Source: three-view drawing plus pictorial views. Frame: mm from the lowest corner of the part. A direction names the side the tool comes from. Give positions to 0.01 mm unless a question says otherwise; leave off trailing zeros. Order: outer loops, then holes, each group sorted by start corner. A loop starts at its lowest first (then second) coordinate and runs counter-clockwise, first axis right, second up. Notation, with made-up numbers: M 74.25,78.5 L 85.25,78.5 A24 ccw 85.25,92.5 Z; hole C -23.75,6.25 d9. An arc over 180 degrees is marked long. Use CSV: the item, a comma, the result in double quotes.
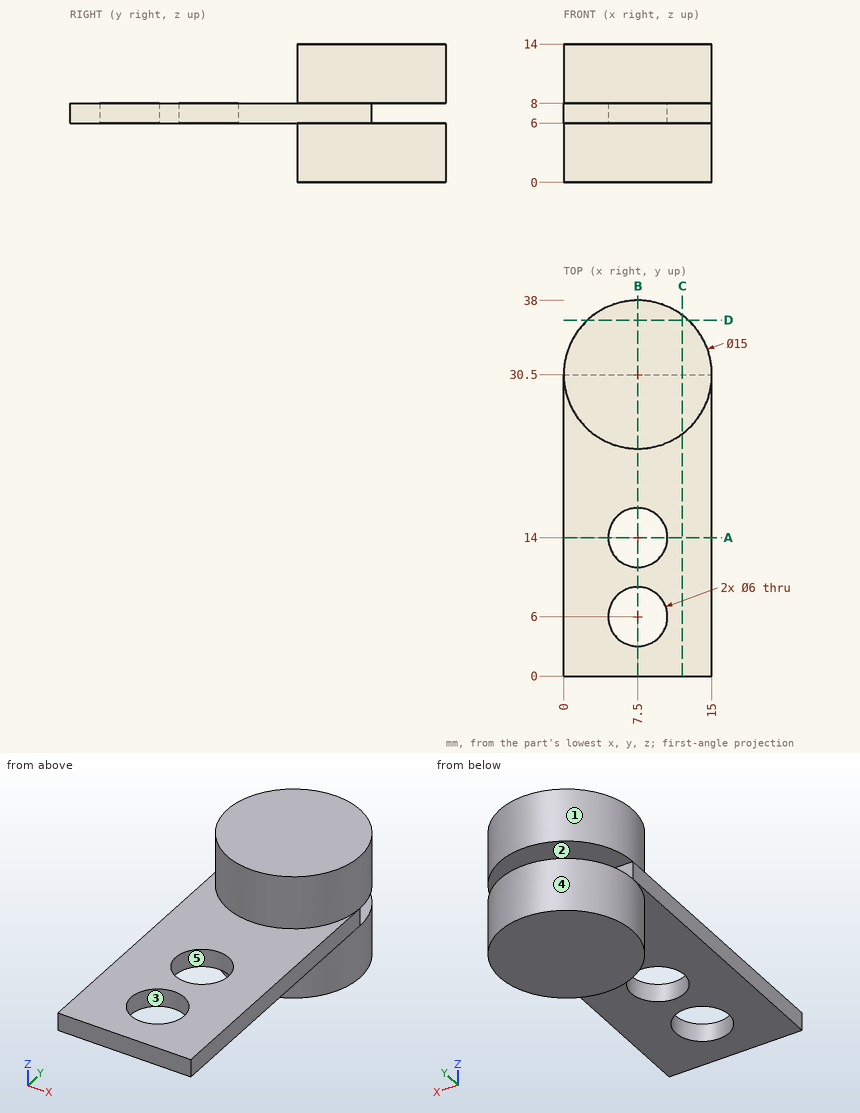
1. Section D-D, the plane y = 36. Return the cut outline in (x, z).
Answer:
outline,"M 2.4,0 L 12.6,0 L 12.6,6 L 2.4,6 Z; M 2.4,8 L 12.6,8 L 12.6,14 L 2.4,14 Z"
2. Section A-A, the plane y = 14. Return the cut outline in (x, z).
Answer:
outline,"M 0,6 L 4.5,6 L 4.5,8 L 0,8 Z; M 10.5,6 L 15,6 L 15,8 L 10.5,8 Z"
3. Pin query (flat end, axial travel): pin 1 Ø1.5 at (x, z) = (8.5, 1.5) entering from -Y; pin 2 Ø8 at (x, z) = (8, 10) entering from +Y; pin 3 Ø5 at (x, z) = (12.5, 7) entering from +Y; pin 4 Ø1 at (x, y) = (11, 6) entering from +Z. Return the tip coordinate at first contact, or that it passes through.
Answer:
pin 1,"y = 23"
pin 2,"y = 38"
pin 3,"y = 37.49"
pin 4,"z = 8"
4. Section C-C, the plane x = 12. Return the cut outline in (y, z), plus the area to 3 significant figures.
Answer:
outline,"M 0,6 L 24.5,6 L 24.5,0 L 36.5,0 L 36.5,6 L 30.5,6 L 30.5,8 L 36.5,8 L 36.5,14 L 24.5,14 L 24.5,8 L 0,8 Z"
area,"205 mm2"
5. Reachability of the marked faces 4 and 5 from +Z, -Z, +X, -X, +Y, -Y: full face, straight path, thin tool, end or side. Return the list, or none.
Answer:
face 4,"-Z"
face 5,"+Z, -Z"
6. Section B-B, the plane x = 7.5. Return the cut outline in (y, z), plus the area to 3 significant figures.
Answer:
outline,"M 0,6 L 3,6 L 3,8 L 0,8 Z; M 9,6 L 11,6 L 11,8 L 9,8 Z; M 17,6 L 23,6 L 23,0 L 38,0 L 38,6 L 30.5,6 L 30.5,8 L 38,8 L 38,14 L 23,14 L 23,8 L 17,8 Z"
area,"217 mm2"
7. Line query: line 1 (Y direction, x = 7.5, z = 7.4); line 2 (Z direction, x = 12.75, y = 31.5); line 3 (Z direction, x = 6.5, y = 18). Output: solid intervals per line, ascending.
Answer:
line 1,"0 to 3, 9 to 11, 17 to 30.5"
line 2,"0 to 6, 8 to 14"
line 3,"6 to 8"
8. Pull-direction query (Y, two-part tool) for the marked faces 1, 2 and 3; classes: +Y half, -Y half, draft (parallel to the pull), parting line (faces both ways), or undercut.
Answer:
face 1,"parting line"
face 2,"draft"
face 3,"undercut"
